Autodesk Inventor part; units mm, degrees
ref_plane "YZ Plane" through (0, 0, 0) normal (1, 0, 0) x (0, 1, 0)
ref_plane "XZ Plane" through (0, 0, 0) normal (0, 1, 0) x (-1, 0, 0)
ref_plane "XY Plane" through (0, 0, 0) normal (0, 0, 1) x (1, 0, 0)
sketch "Sketch1" plane through (0, 0, 0) normal (0, 1, 0) x (-1, 0, 0)
  circle A0 centre (0, 0) radius 1.75
  dimension "d0" = 3.5
extrude "Extrusion1" add sketch "Sketch1" along normal blind 1.7
sketch "Sketch2" plane through (0, 1.7, 0) normal (0, 1, 0) x (1, 0, 0)
  circle A0 centre (0, 0) radius 1
  dimension "d3" = 2
extrude "Extrusion2" add sketch "Sketch2" along normal blind 5.3
thread "Thread1"
fillet "Fillet1" radius 0.4 2 edges at (1.75, 1.7, 0) (1.75, 0, 0)
sketch "Sketch3" plane through (0, 0, 0) normal (0, -1, 0) x (1, 0, 0)
  line L0 (-0.3, -1.75) -> (0.3, -1.75)
  line L1 (0.3, -1.75) -> (0.3, 1.75)
  line L2 (0.3, 1.75) -> (-0.3, 1.75)
  line L3 (-0.3, 1.75) -> (-0.3, -1.75)
  line L4 (-0.3, -1.75) -> (0.3, 1.75) construction
  line L5 (0.3, -1.75) -> (-0.3, 1.75) construction
  circle A0 centre (0, 0) radius 1.75
  point P0 (0.3, -1.7241)
  point P1 (0.3, 1.7241)
  point P2 (-0.3, 1.7241)
  point P3 (-0.3, -1.7241)
  dimension "d9" = 0.6
extrude "Extrusion3" cut sketch "Sketch3" against normal blind 0.6 contours A0 L3 L1
chamfer "Chamfer1" distance 0.2 angle 45 1 edges at (-1, 7, 0)
properties part number "connector_screw" material "Aluminum 6061-AHC"
The listing builds one solid part. Answer for the finished solid, in the listing's coordinates (mm). A direction names the side the tool comes from. Coordinates: 2 decimals unless noted, no trailing zeros. Write each loop counter-clockwise with the first axis right and the second up, starting at its lowest first coordinate (ties: lowest second). Pieces come first, ordered by that corner, then holes. Notation, with made-up numbers: (9.5, 5.25) - (17.5, 5.25) arc R36 ccw to (17.5, 39.25) - close; hole circle Ø4 at (-29.75, 39.5). An arc over 180 degrees is marked (long way). Return JSON: item names as keys, results as strings.
1. Which of the six approach directions +Z, -Z, +X, -X, +Y, -Y give full straight-line access (tool end or side, diameter ignored) to faces 1 (the face through (-0.81, 0.84, 1.55)), 2 (the face through (0, 4, -1))?
Final values:
{"face 1": "+Y, -Y", "face 2": "+Y"}
2. Consider line 1 along Z through (x, y) = (0.6, 2.25); line 2 along Y through (x, z) = (-0.75, -1.15); line 3 along Z through (x, y) = (0, 2.5). Determine where each line is inside the solid, lowest interval first.
Final values:
{"line 1": "-0.8 to 0.8", "line 2": "0 to 1.7", "line 3": "-1 to 1"}
3. The part is cut by section B-B on x = 0. Determine the outline of the cut face in (y, z), then the cut area to 3 significant figures.
Final values:
{"outline": "(0.6, -1.75) - (1.3, -1.75) arc R0.4 ccw to (1.7, -1.35) - (1.7, -1) - (6.8, -1) - (7, -0.8) - (7, 0.8) - (6.8, 1) - (1.7, 1) - (1.7, 1.35) arc R0.4 ccw to (1.3, 1.75) - (0.6, 1.75) - close", "area": "14.3 mm^2"}
4. The part is cut by section A-A on z = 0. Determine the outline of the cut face in (x, y).
Final values:
{"outline": "(-1.75, 0.4) arc R0.4 ccw to (-1.35, 0) - (-0.3, 0) - (-0.3, 0.6) - (0.3, 0.6) - (0.3, 0) - (1.35, 0) arc R0.4 ccw to (1.75, 0.4) - (1.75, 1.3) arc R0.4 ccw to (1.35, 1.7) - (1, 1.7) - (1, 6.8) - (0.8, 7) - (-0.8, 7) - (-1, 6.8) - (-1, 1.7) - (-1.35, 1.7) arc R0.4 ccw to (-1.75, 1.3) - close"}
5. This flat-tipped pin is pushed along its axis until it touches: pin 1 Ø0.5 at (y, z) = (0, 0) entering from -X. Where does it stop, or does it pass through?
Final values:
{"pin 1": "x = -1.72"}
6. The part is cut by section C-C on y = 3.5. Determine the outline of the cut face in (x, z), then the cut area to 3 significant figures.
Final values:
{"outline": "circle Ø2 at (0, 0)", "area": "3.14 mm^2"}
